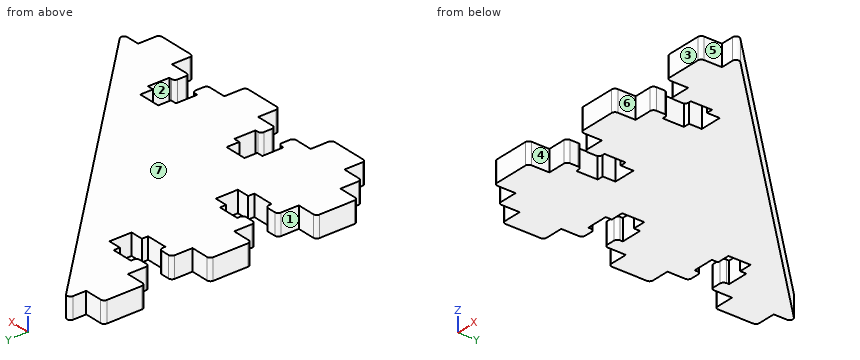
from build123d import *

# Parameters (mm, degrees)
BOSS_EXTRUDE1_DEPTH = 4.95
FILLET1_R           = 0.8


with BuildPart() as part:
    # Sketch2 → Boss-Extrude1 (new body)
    with BuildSketch(Plane.XY):
        Polygon((11.5, 25), (8.5, 25), (8.5, 26.45), (3.5, 26.45), (3.5, 25), (0, 25), (0, 30), (-5, 30), (-5, 39.8), (0, 39.8), (0, 44.8), (3.5, 44.8), (3.5, 43.35), (8.5, 43.35), (8.5, 44.8), (11.5, 44.8), (11.5, 50), (8.5, 50), (8.5, 51.45), (3.5, 51.45), (3.5, 50), (0, 50), (0, 55), (-5, 55), (-5, 64.8), (0, 64.8), (0, 69.8), (69.8, 0), (64.8, 0), (64.8, -5), (55, -5), (55, 0), (50, 0), (50, 3.5), (51.45, 3.5), (51.45, 8.5), (50, 8.5), (50, 11.5), (44.8, 11.5), (44.8, 8.5), (43.35, 8.5), (43.35, 3.5), (44.8, 3.5), (44.8, 0), (39.8, 0), (39.8, -5), (30, -5), (30, 0), (25, 0), (25, 3.5), (26.45, 3.5), (26.45, 8.5), (25, 8.5), (25, 11.5), (19.8, 11.5), (19.8, 8.5), (18.35, 8.5), (18.35, 3.5), (19.8, 3.5), (19.8, 0), (14.8, 0), (14.8, -5), (5, -5), (5, 0), (0, 0), (0, 5), (-5, 5), (-5, 14.8), (0, 14.8), (0, 19.8), (3.5, 19.8), (3.5, 18.35), (8.5, 18.35), (8.5, 19.8), (11.5, 19.8), align=None)
    extrude(amount=BOSS_EXTRUDE1_DEPTH)

    # Fillet1
    fillet1_edges = [part.edges().sort_by_distance(p)[0] for p in [
        (19.8, 3.5, 2.475),
        (19.8, 0, 2.475),
        (14.8, -5, 2.475),
        (5, -5, 2.475),
        (0, 0, 2.475),
        (-5, 5, 2.475),
        (-5, 14.8, 2.475),
        (0, 19.8, 2.475),
        (3.5, 19.8, 2.475),
        (3.5, 25, 2.475),
        (0, 25, 2.475),
        (-5, 30, 2.475),
        (-5, 39.8, 2.475),
        (0, 44.8, 2.475),
        (3.5, 44.8, 2.475),
        (3.5, 50, 2.475),
        (0, 50, 2.475),
        (-5, 55, 2.475),
        (-5, 64.8, 2.475),
        (0, 69.8, 2.475),
        (69.8, 0, 2.475),
        (64.8, -5, 2.475),
        (55, -5, 2.475),
        (50, 0, 2.475),
        (50, 3.5, 2.475),
        (44.8, 3.5, 2.475),
        (44.8, 0, 2.475),
        (39.8, -5, 2.475),
        (30, -5, 2.475),
        (25, 0, 2.475),
        (25, 3.5, 2.475),
    ]]
    fillet(fillet1_edges, radius=FILLET1_R)


solid = part.part
Read the model definition and answer for the solid it produces. Units are mm, in the model's axes. Face numbers are marked on the shaded views. A direction names the side the tool comes from. Round coordinates to 2 decimals unless told otherwise and drop trailing zeros. Write each loop counter-clockwise with the first axis right and the second up, starting at its lowest first coordinate (ties: lowest second). Pieces come first, ordered by that corner, then holes.
Q1. Find section A-A on x = 10. Determine the outline of the cut face in (y, z), and give its area (3 significant figures).
Values:
outline: (-5, 0) - (19.8, 0) - (19.8, 4.95) - (-5, 4.95) - close; (25, 0) - (44.8, 0) - (44.8, 4.95) - (25, 4.95) - close; (50, 0) - (59.8, 0) - (59.8, 4.95) - (50, 4.95) - close
area: 269 mm2
Q2. Straight lines are drawn through the part: line 1 (X direction, y = -1, z = 1.5); line 2 (X direction, y = 1, z = 0.9); line 3 (X direction, y = 19, z = 4.75). For each, find the intervals that lie inside material, in ascending order.
Values:
line 1: x = 5 to 14.8, 30 to 39.8, 55 to 64.8
line 2: x = 0 to 19.8, 25 to 44.8, 50 to 68.64
line 3: x = 0 to 3.5, 8.5 to 50.8
Q3. Flat-ended cylindrical pins translate along their axes: P1, Ø2, axis at x = 2, z = 2, coming from the +Y side; P2, Ø1.6, axis at x = 44, z = 3.5, coming from the -Y side; P3, Ø1, axis at x = 2, z = 3.5, coming from the +Y side. Find the tip coordinate at first contact, or state that the pin passes through.
Values:
P1: stops at y = 68.64
P2: stops at y = 0
P3: stops at y = 68.3
Q4. A tool of negligible diameter and unlimited length cuts with its end or side. For the marked faces 1, 2, 3 and 4, from which of +Z, -Z, +X, -X, +Y, -Y can it reach the whole face along a straight path? Write none if from no direction.
Values:
face 1: +Z, -Z, -X
face 2: +Z, -Z
face 3: +Z, -Z, +X, -X, -Y
face 4: +Z, -Z, -Y
Q5. Find section C-C on x = 62.5. Determine the outline of the cut face in (y, z).
Values:
outline: (-5, 0) - (7.3, 0) - (7.3, 4.95) - (-5, 4.95) - close
Q6. Find section B-B on y = 41. Determine the outline of the cut face in (x, z).
Values:
outline: (0, 0) - (28.8, 0) - (28.8, 4.95) - (0, 4.95) - close
Q7. The mould has two halves that part along X. Classify the marked faces 5, 6 and 7: released by +X, released by -X, zero draft, split by the parting line, or undercut.
Values:
face 5: released by +X
face 6: undercut
face 7: zero draft
